The listing builds one solid part. Answer for the finished solid, in the listing's coordinates (mm). Face numbers are marked on the shaded views. A direction names the side the tool comes from. Round coordinates to 2 decimals unless told otherwise and drop trailing zeros. Write each loop counter-clockwise with the first axis right and the second up, starting at its lowest first coordinate (ties: lowest second). Pieces come first, ordered by that corner, then holes. Notation, with made-up numbers: (-38.5, 29) - (-6.5, 29) arc R27 cw to (-6.5, 55) - close; hole circle Ø11 at (17.5, 29.25). An arc over 180 degrees is marked (long way). Return JSON: item names as keys, results as strings. Group by question number.
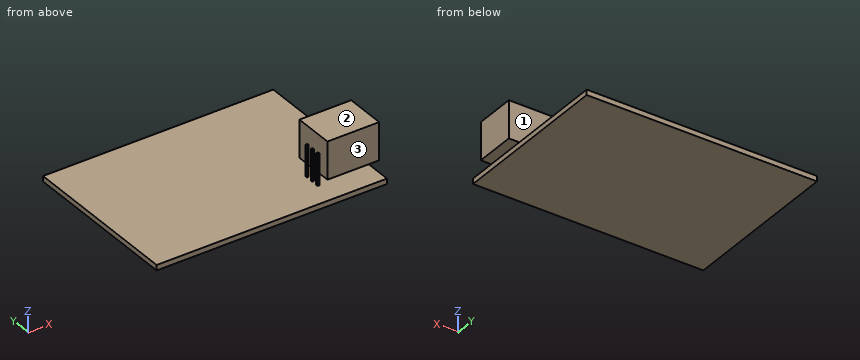
from build123d import *

# Parameters (mm, degrees)
F0_W     = 75.184
F0_H     = 53.594
F1_DEPTH = 1.7272
F2_W     = 16.891
F2_H     = 13.208
F3_DEPTH = 12.192
F4_W     = 0.635
F4_H     = 0.635
F5_DEPTH = 10.16


with BuildPart() as f1:
    # F0 (on Top) → F1 (new body)
    with BuildSketch(Plane.XY):
        with Locations((37.592, 26.797)):
            Rectangle(F0_W, F0_H)
    extrude(amount=F1_DEPTH)

    # F2 (on face) → F3 (join)
    with BuildSketch(Plane.XY.offset(1.7272)):
        with Locations((70.1675, 15.24)):
            Rectangle(F2_W, F2_H)
    extrude(amount=F3_DEPTH)

    # F4 (on face) → F5 (join)
    with BuildSketch(Plane.XY.offset(1.7272)):
        with Locations((58.1025, 7.9375)):
            Rectangle(F4_W, F4_H)
        with Locations((58.1025, 10.4775)):
            Rectangle(F4_W, F4_H)
        with Locations((58.1025, 13.0175)):
            Rectangle(F4_W, F4_H)
    extrude(amount=F5_DEPTH)


solid = f1.part
(1) Find section C-C (x = 49). Write down the section's boundary in (y, z), plus the area to 3 significant figures.
(2) Find section A-A (z = 6.75). Write down the section's boundary in (x, y) (3 decimals), plus the area to 3 significant figures.
(3) Consider line 1 (X direction, y = 10.5, z = 8.75) (3 decimals); line 2 (Z direction, x = 61, y = 11); line 3 (X direction, y = 15.5, z = 8.5). Determine where each line is inside the solid, lowest interval first.
(4) Find section D-D (y = 31). Write down the section's boundary in (x, z), plus the area to 3 significant figures.
(5) Find section B-B (y = 18). Write down the section's boundary in (x, z), plus the area to 3 significant figures.
(6) Flat-ended cylindrical pins translate along their axes: pin 1 (0.7 mm diameter, centred on x = 58, y = 13, fed in from +Z); pin 2 (3.5 mm diameter, centred on y = 18, z = 10, fed in from -X); pin 3 (3.5 mm diameter, centred on x = 69.5, z = 9, fed in from +Y). Find the tip coordinate at first contact, or state that the pin passes through.
(7) For the marked faces 1, 2 and 3, determine the directions among +Z, -Z, +X, -X, +Y, -Y from which every point of the face is accessible in a straight line to the end or side of a thin tool.
Check sheet entries:
{
 "1": {"outline": "(0, 0) - (53.59, 0) - (53.59, 1.73) - (0, 1.73) - close", "area": "92.6 mm^2"},
 "2": {"outline": "(57.785, 7.62) - (58.42, 7.62) - (58.42, 8.255) - (57.785, 8.255) - close; (57.785, 10.16) - (58.42, 10.16) - (58.42, 10.795) - (57.785, 10.795) - close; (57.785, 12.7) - (58.42, 12.7) - (58.42, 13.335) - (57.785, 13.335) - close; (61.722, 8.636) - (78.613, 8.636) - (78.613, 21.844) - (61.722, 21.844) - close", "area": "224 mm^2"},
 "3": {"line 1": "x = 57.785 to 58.42, 61.722 to 78.613", "line 2": "z = 0 to 1.73", "line 3": "x = 61.72 to 78.61"},
 "4": {"outline": "(0, 0) - (75.18, 0) - (75.18, 1.73) - (0, 1.73) - close", "area": "130 mm^2"},
 "5": {"outline": "(0, 0) - (75.18, 0) - (75.18, 1.73) - (78.61, 1.73) - (78.61, 13.92) - (61.72, 13.92) - (61.72, 1.73) - (0, 1.73) - close", "area": "336 mm^2"},
 "6": {"pin 1": "stops at z = 11.89", "pin 2": "stops at x = 61.72", "pin 3": "stops at y = 21.84"},
 "7": {"face 1": "+Z, +X, -X, +Y", "face 2": "+Z, +X, -X, +Y, -Y", "face 3": "+Z, +X, -X, -Y"}
}
